Part model, mm, in its own coordinate system. A direction names the side the tool comes from. Coordinates: 2 decimals unless noted, no trailing zeros. Write each loop counter-clockwise with the first axis right and the second up, starting at its lowest first coordinate (ties: lowest second). Pieces come first, ordered by that corner, then holes. Notation, with made-up numbers: (-35.5, 86.5) - (-21.5, 86.5) arc R4 cw to (-21.5, 93.5) - close; hole circle Ø7 at (81.25, 56). An arc over 180 degrees is marked (long way). Use one line per item in the form item = value. Start each with the question number.
from build123d import *

# Parameters (mm, degrees)
F2_SIZE = 5


with BuildPart() as f1:
    # F0 (on Front) → F1 (revolve)
    with BuildSketch(Plane.XZ):
        Polygon((-25, 0), (-13.5, 0), (-13.5, 40), (-16, 40), (-16, 35.1), (-15, 33.9), (-16, 25.9), (-15, 24.7), (-16, 16.7), (-15, 15.5), (-16, 7.5), (-21.5, 2), (-25, 2), align=None)
    revolve(axis=Axis((0, 0, -0.481866), (0, 0, -1)))

    # F2
    f2_edges = [f1.edges().sort_by_distance(p)[0] for p in [
        (13.5, 0, 0),
    ]]
    chamfer(f2_edges, length=F2_SIZE)


solid = f1.part
Q1. Pin check, flat tips, straight feed: P1, Ø2, axis at y = 2, z = 7, coming from the -X side; P2, Ø3, axis at x = 8.5, y = -9.5, coming from the +Z side; P3, Ø1, axis at y = 3.5, z = 14.5, coming from the +X side; P4, Ø3, axis at y = 0, z = 17, coming from the -X side. Stop position of each tip, or through.
Q2. Mould opens along Z. For faces 4 (the conical face through (3.313, -14.921, 31.622)), 5 (the flat face through (0, 19, 0)), 6 (the cylindrical face through (3.47, -15.62, 37.52)), 7 (the conical face through (3.313, -14.921, 13.222)) say: released by +Z, released by -Z, zero draft, split by the parting line, or undercut.
Q3. Slice it at A-A (x = 0). List the corners of the cut face in (y, z).
Q4. Which spindle directions (+Z, -Z, +X, -X, +Y, -Y) get a long thin tool onto all of the face, cutting with end or side? Do faces 1 (the cylindrical face through (2.93, -13.18, 22.74)), 2 (the flat face through (11, 19, 2)), 3 (the conical face through (3.313, -14.921, 22.422)). Say none if no direction does.
Q5. Drill centre lines: probe 1 along Y at (x, z) = (0, 26); probe 2 along X at (y, z) = (-6, 22); probe 3 along Y at (x, z) = (0, 25). Where is each one in solid material? Low to high.
Q6. Slice it at D-D (x = 15). Count the separate pieces of the cut face and the enclosed holes in it, plus the area to 3 significant figures.
Q7. Slice it at C-C (z = 17.5). List the corners of the cut face in (x, y).
Solution:
q1.P1 = -17.39
q1.P2 = 40
q1.P3 = 14.84
q1.P4 = -16
q2.face_4 = undercut
q2.face_5 = released by -Z
q2.face_6 = zero draft
q2.face_7 = undercut
q3.outline = (-25, 0) - (-18.5, 0) - (-13.5, 5) - (-13.5, 40) - (-16, 40) - (-16, 35.1) - (-15, 33.9) - (-16, 25.9) - (-15, 24.7) - (-16, 16.7) - (-15, 15.5) - (-16, 7.5) - (-21.5, 2) - (-25, 2) - close; (13.5, 5) - (18.5, 0) - (25, 0) - (25, 2) - (21.5, 2) - (16, 7.5) - (15, 15.5) - (16, 16.7) - (15, 24.7) - (16, 25.9) - (15, 33.9) - (16, 35.1) - (16, 40) - (13.5, 40) - close
q4.face_1 = +Z, -Z
q4.face_2 = +Z
q4.face_3 = none
q5.probe_1 = -15.99 to -13.5, 13.5 to 15.99
q5.probe_2 = -14.12 to -12.09, 12.09 to 14.12
q5.probe_3 = -15.25 to -13.5, 13.5 to 15.25
q6.separate_pieces = 4
q6.enclosed_holes = 0
q6.area = 410 mm2
q7.outline = circle Ø31.8 at (0, 0); hole circle Ø27 at (0, 0)
